Autodesk Inventor part; units mm, degrees
ref_plane "YZ Plane" through (0, 0, 0) normal (1, 0, 0) x (0, 1, 0)
ref_plane "XZ Plane" through (0, 0, 0) normal (0, 1, 0) x (-1, 0, 0)
ref_plane "XY Plane" through (0, 0, 0) normal (0, 0, 1) x (1, 0, 0)
sketch "Sketch1" plane through (0, 0, 0) normal (0, 0, 1) x (1, 0, 0)
  line L0 (0, 0) -> (35, 0)
  line L1 (35, 0) -> (35, -17.5)
  line L2 (35, -17.5) -> (0, -17.5)
  line L3 (0, -17.5) -> (0, 0)
  dimension "d0" = 17.5
  dimension "d1" = 35
extrude "Extrusion1" add sketch "Sketch1" against normal blind 2.8
sketch "Sketch2" plane through (0, 0, 0) normal (0, 0, 1) x (1, 0, 0)
  line L0 (35, -17.5) -> (0, -17.5)
  line L1 (5.75, -23.2591) -> (29.25, -23.2591)
  line L2 (29.25, -23.2591) -> (29.25, -5.5)
  line L3 (29.25, -5.5) -> (5.75, -5.5)
  line L4 (5.75, -5.5) -> (5.75, -23.2591)
  point P0 (17.5, -5.5)
  point P1 (17.5, -17.5)
  dimension "d4" = 12
  dimension "d5" = 23.5
extrude "Extrusion2" cut sketch "Sketch2" against normal through all
sketch "Sketch3" plane through (0, 0, 0) normal (0, 0, 1) x (1, 0, 0)
  line L0 (0, 0) -> (35, 0)
  line L1 (0, -17.5) -> (0, 0)
  point P0 (8, -2.4)
  point P1 (27, -2.4)
  dimension "d8" = 8
  dimension "d9" = 19
  dimension "d10" = 2.4
hole "Hole1" at (8, -2.4, 0) at (27, -2.4, 0) direction (0, 0, -1) diameter 2.2 end through all
sketch "Sketch4" plane through (0, 0, 0) normal (0, 0, 1) x (1, 0, 0)
  line L0 (29.25, -5.5) -> (29.25, -17.5)
  line L1 (5.75, -17.5) -> (0, -17.5)
  line L2 (5.75, -17.5) -> (5.75, -5.5)
  point P0 (2.875, -11.5)
  point P1 (31.875, -11.5)
  point P2 (5.75, -11.5)
  point P3 (29.25, -11.5)
  point P4 (2.875, -17.5)
hole "Hole2" at (2.875, -11.5, 0) at (31.875, -11.5, 0) direction (0, 0, -1) diameter 1.567 end through all
properties part number "Servo Mount2"
Model file for the job. Use its own axes, mm. A direction names the side the tool comes from. Round coordinates to 2 decimals unless told otherwise and drop trailing zeros. Order: outer loops, then holes, each group sorted by start corner. A loop starts at its lowest first (then second) coordinate and runs counter-clockwise, first axis right, second up.
(1) Band-saw the part on B-B (y = -11.5). List the corners of the cut face in (x, z).
(2) Pull direction X, two halves, no side cores. Call faces 3 (the face through (17, 0, -1)), 4 (the face through (32.64, -11.33, -1.42)), 5 (the face through (35, -9, -1)), 6 (the face through (29.25, -12, -1)): released by +X, released by -X, zero draft, split by the parting line, or undercut.
(3) Band-saw the part on C-C (y = -7.25). List the corners of the cut face in (x, z).
(4) 3-axis set-ups, long thin cutter, end or side, ignore diameter. For faces 1 (the face through (18, -5.5, -1)), 2 (the face through (0, -9, -1)): which of +Z, -Z, +X, -X, +Y, -Y reach the whole face in a straight line?
(5) Pin check, flat tips, straight feed: pin 1 (1.4 mm diameter, centred on x = 31.875, y = -11.5, fed in from +Z); pin 2 (0.8 mm diameter, centred on x = 20.5, z = -0.5, fed in from -Y). Stop position of each tip, or through.
(6) Drill centre lines: line 1 (X direction, y = -2.4, z = -0.8); line 2 (X direction, y = -11.5, z = -1.05); line 3 (X direction, y = -9.75, z = -0.5). Where is each one in solid material? Low to high.
(7) Band-saw the part on A-A (x = 8). List the corners of the cut face in (y, z).
(8) Band-saw the part on D-D (y = -2.4). List the corners of the cut face in (x, z), then the cut area to 3 significant figures.
Verdict:
1. outline: (0, -2.8) - (2.09, -2.8) - (2.09, 0) - (0, 0) - close; (3.66, -2.8) - (5.75, -2.8) - (5.75, 0) - (3.66, 0) - close; (29.25, -2.8) - (31.09, -2.8) - (31.09, 0) - (29.25, 0) - close; (32.66, -2.8) - (35, -2.8) - (35, 0) - (32.66, 0) - close
2. face 3: zero draft
2. face 4: undercut
2. face 5: released by +X
2. face 6: undercut
3. outline: (0, -2.8) - (5.75, -2.8) - (5.75, 0) - (0, 0) - close; (29.25, -2.8) - (35, -2.8) - (35, 0) - (29.25, 0) - close
4. face 1: +Z, -Z, -Y
4. face 2: +Z, -Z, -X, +Y, -Y
5. pin 1: passes through
5. pin 2: stops at y = -5.5
6. line 1: x = 0 to 6.9, 9.1 to 25.9, 28.1 to 35
6. line 2: x = 0 to 2.09, 3.66 to 5.75, 29.25 to 31.09, 32.66 to 35
6. line 3: x = 0 to 5.75, 29.25 to 35
7. outline: (-5.5, -2.8) - (-3.5, -2.8) - (-3.5, 0) - (-5.5, 0) - close; (-1.3, -2.8) - (0, -2.8) - (0, 0) - (-1.3, 0) - close
8. outline: (0, -2.8) - (6.9, -2.8) - (6.9, 0) - (0, 0) - close; (9.1, -2.8) - (25.9, -2.8) - (25.9, 0) - (9.1, 0) - close; (28.1, -2.8) - (35, -2.8) - (35, 0) - (28.1, 0) - close
8. area: 85.7 mm2
